Autodesk Inventor part; units mm, degrees
ref_plane "YZ Plane" through (0, 0, 0) normal (1, 0, 0) x (0, 1, 0)
ref_plane "XZ Plane" through (0, 0, 0) normal (0, 1, 0) x (-1, 0, 0)
ref_plane "XY Plane" through (0, 0, 0) normal (0, 0, 1) x (1, 0, 0)
sketch "Sketch1" plane through (0, 0, 0) normal (0, 0, 1) x (1, 0, 0)
  line L0 (0, 0) -> (52, 0)
  line L1 (52, 0) -> (52, 25)
  line L2 (52, 25) -> (0, 25)
  line L3 (0, 25) -> (0, 0)
  line L4 (11, 0) -> (41, 0)
  line L5 (41, 0) -> (41, -3)
  line L6 (41, -3) -> (11, -3)
  line L7 (11, -3) -> (11, 0)
  line L8 (0, 5) -> (-3, 5)
  line L9 (-3, 5) -> (-3, 15)
  line L10 (-3, 15) -> (0, 15)
  line L11 (0, 15) -> (0, 5)
  line L12 (26, 25) -> (26, 0)
  line L13 (52, 5) -> (55, 5)
  line L14 (55, 5) -> (55, 15)
  line L15 (55, 15) -> (52, 15)
  point P0 (0, 15)
  point P1 (41, 0)
  point P2 (52, 5)
  point P3 (0, 15)
  dimension "d0" = 52
  dimension "d1" = 30
  dimension "d2" = 3
  dimension "d3" = 25
  dimension "d4" = 3
  dimension "d5" = 10
  dimension "d6" = 5
extrude "Plate1" add sketch "Sketch1" along normal blind 3
equation "\"d0\" = A_width + 2 * A_joint_tolerance"
equation "\"d2\" = plate_thickness"
equation "\"d4\" = plate_thickness"
equation "\"d7\" = Thickness"
equation "\"Thickness\" = plate_thickness"
equation "\"BendRadius\" = Thickness"
equation "\"BendReliefWidth\" = Thickness"
equation "\"BendReliefDepth\" = 0.5 * Thickness"
equation "\"CornerReliefSize\" = 4 * Thickness"
equation "\"MinimumRemnant\" = 2 * Thickness"
equation "\"TransitionRadius\" = BendRadius"
equation "\"JacobiRadiusSize\" = BendRadius"
equation "\"GapSize\" = Thickness"
equation "\"A_width\" = 46"
equation "\"A_joint_diameter\" = 16"
equation "\"l___________\" = 0"
equation "\"l__________\" = 0"
equation "\"l_________\" = 0"
equation "\"rivet_diameter\" = 3.35"
equation "\"plate_thickness\" = 3"
equation "\"l________\" = 0"
equation "\"A_joint_tolerance\" = 3"
equation "\"A_B_spacing\" = 2"
equation "\"L_Piston_Bottom\" = 21"
equation "\"L_Piston_Top\" = 25"
equation "\"thin_plate\" = 1.5"
properties part number "bottom_hinge_002" material "Stainless Steel"
Model file for the job. Use its own axes, mm. A direction names the side the tool comes from. Give positions to 0.01 mm unless a question says otherwise; leave off trailing zeros. Order: outer loops, then holes, each group sorted by start corner. A loop starts at its lowest first (then second) coordinate and runs counter-clockwise, first axis right, second up. Notation, with made-up numbers: (10.5, -3.5) - (65.5, -3.5) arc R14 ccw to (65.5, 17.5) - close; hole circle Ø9 at (-17, 37.5). An arc over 180 degrees is marked (long way). Return JSON: item names as keys, results as strings.
1) 3-axis set-ups, long thin cutter, end or side, ignore diameter. For faces 1 (the flat face through (0, 3, 1)), 2 (the flat face through (52, 20, 1)), 3 (the flat face through (26, 11, 0)), 4 (the flat face through (52, 2, 1)), 5 (the flat face through (-2, 15, 1)): which of +Z, -Z, +X, -X, +Y, -Y reach the whole face in a straight line?
Geometry says:
{"face 1": "+Z, -Z, -X, -Y", "face 2": "+Z, -Z, +X, +Y", "face 3": "-Z, +X, -X, +Y, -Y", "face 4": "+Z, -Z, +X, -Y", "face 5": "+Z, -Z, -X, +Y"}
2) Cut at C-C, the plane x = 5. Give the cut face in (y, z), plus the area to 3 significant figures.
Geometry says:
{"outline": "(0, 0) - (25, 0) - (25, 3) - (0, 3) - close", "area": "75.0 mm²"}
3) Flat gauge pins, fed straight in: P1, Ø0.9, axis at y = 19, z = 1.5, coming from the -X side; P2, Ø1.5, axis at y = 21, z = 1, coming from the +X side; P3, Ø1.5, axis at x = 4, z = 1, coming from the -Y side. Where does each tip first touch, or does it go through?
Geometry says:
{"P1": "x = 0", "P2": "x = 52", "P3": "y = 0"}
4) Cut at A-A, the plane z = 1.35. Give the cut face in (x, y), plus the area to 3 significant figures.
Geometry says:
{"outline": "(-3, 5) - (0, 5) - (0, 0) - (11, 0) - (11, -3) - (41, -3) - (41, 0) - (52, 0) - (52, 5) - (55, 5) - (55, 15) - (52, 15) - (52, 25) - (0, 25) - (0, 15) - (-3, 15) - close", "area": "1,450 mm²"}
5) Probe line 1 (Y direction, x = 44, z = 0.35); line 2 (X direction, y = 17.25, z = 1.9); line 3 (X direction, y = -1.5, z = 1.15). List the from-to ranges inside material, lowest first. Write a range as from..to.
Geometry says:
{"line 1": "0..25", "line 2": "0..52", "line 3": "11..41"}
6) Cut at B-B, the plane y = 3.25. Give the cut face in (x, z).
Geometry says:
{"outline": "(0, 0) - (52, 0) - (52, 3) - (0, 3) - close"}
